Could you check a few things on this model? Use its own coordinates, in mm. Coordinates: 2 decimals unless noted, no trailing zeros. Write each loop counter-clockwise with the first axis right and the second up, starting at its lowest first coordinate (ties: lowest second). Pieces come first, ordered by that corner, then holes.
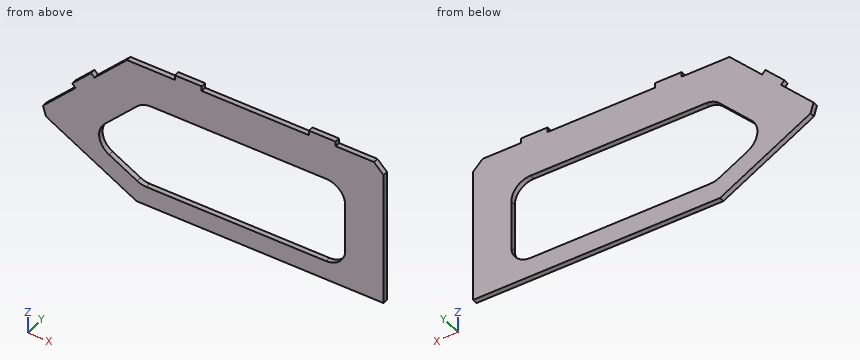
```python
from build123d import *

# Parameters (mm, degrees)
F1_DEPTH = 3.429


# Not quite as in the source:
# - ends of sketch curves that miss each other by under 0.0002 mm in the source are joined


with BuildPart() as f1:
    # F0 (on Front) → F1 (new body)
    with BuildSketch(Plane.XZ):
        Polygon((-357.469059, -352.4197422), (-375.249059, -352.4197422), (-375.249059, -355.5947422), (-406.999059, -355.5947422), (-428.5679516, -377.1636348), (-430.8130322, -374.9185542), (-443.3853718, -387.4909192), (-441.1403166, -389.7359998), (-462.7092092, -411.3048924), (-460.7568382, -417.970716), (-400.649059, -450.8447422), (-236.819059, -450.8447422), (-236.819059, -361.9447422), (-243.169059, -355.5947422), (-268.569059, -355.5947422), (-268.569059, -352.4197422), (-286.349059, -352.4197422), (-286.349059, -355.5947422), (-357.469059, -355.5947422), align=None)
        with BuildLine():
            ThreePointArc((-418.8754328238, -426.4010670387), (-425.3527857587, -417.0618193312), (-421.7617140211, -406.2784129789))
            Line((-421.7617140211, -406.2784129789), (-400.1977772, -384.7144706))
            ThreePointArc((-400.1977772, -384.7144706), (-396.0776022944, -381.9614687005), (-391.217531, -380.9947422))
            Line((-391.217531, -380.9947422), (-274.919059, -380.9947422))
            ThreePointArc((-274.919059, -380.9947422), (-265.9388028789, -384.7144860789), (-262.219059, -393.6947422))
            Line((-262.219059, -393.6947422), (-262.219059, -425.4447422))
            ThreePointArc((-262.219059, -425.4447422), (-265.9388028789, -434.4249983211), (-274.919059, -438.1447422))
            Line((-274.919059, -438.1447422), (-394.1569714, -438.1447422))
            ThreePointArc((-394.1569714, -438.1447422), (-397.3019244332, -437.7491832852), (-400.250969717, -436.5871469904))
            Line((-400.250969717, -436.5871469904), (-418.8754328238, -426.4010670387))
        make_face(mode=Mode.SUBTRACT)
    extrude(amount=F1_DEPTH)


solid = f1.part
```
1. I want a section at C-C on x = -280. Please give me the cut outline in (y, z), plus the area to 3 significant figures.
Verdict:
outline: (-3.43, -450.84) - (0, -450.84) - (0, -438.14) - (-3.43, -438.14) - close; (-3.43, -380.99) - (0, -380.99) - (0, -352.42) - (-3.43, -352.42) - close
area: 142 mm2
2. Please list where these lines run through material, in increasing order: line 1 along Z through (x, y) = (-332, -1.85); line 2 along Z through (x, y) = (-274.5, -2.7); line 3 along X through (y, z) = (-1.6, -384).
Verdict:
line 1: z = -450.84 to -438.14, -380.99 to -355.59
line 2: z = -450.84 to -438.14, -381 to -352.42
line 3: x = -439.89 to -399.42, -266.72 to -236.82
3. I want a section at D-D on z = -359. Please give me the cut outline in (x, y).
Verdict:
outline: (-410.4, -3.43) - (-239.76, -3.43) - (-239.76, 0) - (-410.4, 0) - close
4. For pin 1 (2 mm diameter, centred on x = -321, y = -2, fed in from +Z); pin 2 (1 mm diameter, centred on y = -2, z = -354.5, fed in from +X), each with a flat end and sliding along its axis, tell me the tip position at first contact or that it passes through.
Verdict:
pin 1: stops at z = -355.59
pin 2: stops at x = -268.57
5. I want a section at B-B on x = -316.5. Please give me the cut outline in (y, z).
Verdict:
outline: (-3.43, -450.84) - (0, -450.84) - (0, -438.14) - (-3.43, -438.14) - close; (-3.43, -380.99) - (0, -380.99) - (0, -355.59) - (-3.43, -355.59) - close
